Read the model definition and answer for the solid it produces. Units are mm, in the model's axes. A direction names the side the tool comes from. Round coordinates to 2 decimals unless told otherwise and drop trailing zeros. Order: outer loops, then holes, each group sorted by start corner. A loop starts at its lowest first (then second) coordinate and runs counter-clockwise, first axis right, second up. Notation, with made-up numbers: (-36.75, 10.5) -> (-8.75, 10.5) arc R10 ccw to (-8.75, 28.5) -> close; hole circle Ø2 at (30, -14). An arc over 180 degrees is marked (long way). Answer as a JSON object with one key per item and string values. Group by question number.
Item 1: Consider probe 1 along Z at (x, y) = (-2, -58.5); probe 2 along X at (y, z) = (1, 16.5); probe 3 along Y at (x, z) = (4, 20.5). Determine where each line is inside the solid, lowest interval first. Write a range as from..to.
Item 2: Section A-A, the plane y = 0 is taken. Write down the section's boundary in (x, z).
Item 3: Section C-C, the plane z = -12.5 is taken. Write down the section's boundary in (x, y).
Item 4: Given P1, Ø3, axis at y = 7.5, z = 32.5, coming from the -X side; P2, Ø12, axis at y = 32.5, z = 22.5, coming from the +X side; P3, Ø1, axis at x = -45, z = 16, coming from the +Y side, each flat-ended and moving along its own axis, determine where each tip first touches the part or whether it passes through.
Item 5: For faces 1 (the cylindrical face through (-7.39, 33.28, -20.66)), 2 (the flat face through (1, 1, 43.406)), determine the directions among +Z, -Z, +X, -X, +Y, -Y from which every point of the face is accessible in a straight line to the end or side of a thin tool.
from build123d import *

# Parameters (mm, degrees)
F0_W     = 74.031934
F0_H     = 43.405589
F2_R     = 34.091138
F3_DEPTH = 41.91
F4_R     = 10.16


with BuildPart() as f1:
    # F0 (on Front) → F1 (revolve)
    with BuildSketch(Plane.XZ):
        with Locations((37.015967, 21.702794)):
            Rectangle(F0_W, F0_H)
    revolve(axis=Axis((0, 0, 21.702794), (0, 0, 1)))

    # F2 (on face) → F3 (join)
    with BuildSketch(Plane(origin=(0, 0, 0), x_dir=(1, 0, 0), z_dir=(0, 0, -1))):
        Circle(F2_R)
    extrude(amount=F3_DEPTH)

    # F4
    f4_edges = [f1.edges().sort_by_distance(p)[0] for p in [
        (-74.031934, 0, 43.405589),
    ]]
    fillet(f4_edges, radius=F4_R)


solid = f1.part
Values found:
{
 "1": {"probe 1": "0..43.41", "probe 2": "-74.03..74.03", "probe 3": "-73.92..73.92"},
 "2": {"outline": "(-74.03, 0) -> (-34.09, 0) -> (-34.09, -41.91) -> (34.09, -41.91) -> (34.09, 0) -> (74.03, 0) -> (74.03, 33.25) arc R10.16 ccw to (63.87, 43.41) -> (-63.87, 43.41) arc R10.16 ccw to (-74.03, 33.25) -> close"},
 "3": {"outline": "circle Ø68.18 at (0, 0)"},
 "4": {"P1": "x = -73.79", "P2": "x = 69.13", "P3": "y = 59.16"},
 "5": {"face 1": "-Z", "face 2": "+Z, +X, -X, +Y, -Y"}
}
